Source: CAD feature listing. Evaluate the final solid. Frame: model axes, mm. A direction names the side the tool comes from. Give positions to 0.01 mm unless a question says otherwise; leave off trailing zeros. Loops run counter-clockwise (first coordinate to the right, second up) from the corner with the lowest first, then second, coordinate; pieces in that order, holes last. Notation, with made-up numbers: M 14,-31 L 25,-31 A24 cw 25,6 Z; hole C 35,-32 d2. An arc over 180 degrees is marked long. Answer in a Markdown table with one row per item.
```python
from build123d import *

# Parameters (mm, degrees)
F0_W     = 10
F0_H     = 75
F1_DEPTH = 12.5
F2_R     = 5
F3_DEPTH = 400.001
F4_R     = 5
F5_DEPTH = 50
F6_R     = 20
F7_R     = 3
F8_DEPTH = 140.9584442942


with BuildPart() as f1:
    # F0 (on Front) → F1 (new body, symmetric)
    with BuildSketch(Plane.XZ):
        Polygon((129.7779953739, 41.1399305532), (-70.2220046261, 41.1399305532), (-70.2220046261, 25.182486259), (-60.2220046261, 25.182486259), (129.7779953739, 25.182486259), align=None)
        Polygon((329.7779953739, 41.1399305532), (129.7779953739, 41.1399305532), (129.7779953739, 25.182486259), (319.7779953739, 25.182486259), (329.7779953739, 25.182486259), align=None)
        with Locations((-65.2220046261, -12.317513741)):
            Rectangle(F0_W, F0_H)
        with Locations((324.7779953739, -12.317513741)):
            Rectangle(F0_W, F0_H)
    extrude(amount=F1_DEPTH, both=True)

    # F2 (on face) → F3 (cut, through all)
    with BuildSketch(Plane(origin=(-70.2220046261, 0, 0), x_dir=(0, -1, 0), z_dir=(-1, 0, 0))):
        with Locations((0, -29.817513741)):
            Circle(F2_R)
    extrude(amount=-F3_DEPTH, mode=Mode.SUBTRACT)

    # F4 (on face) → F5 (join)
    with BuildSketch(Plane.XY.offset(41.1399305532)):
        with Locations((129.7779953739, 0)):
            Circle(F4_R)
    extrude(amount=F5_DEPTH)

    # F6
    f6_edges = [f1.edges().sort_by_distance(p)[0] for p in [
        (-60.222005, 0, 25.182486),
        (319.777995, 0, 25.182486),
    ]]
    fillet(f6_edges, radius=F6_R)

    # F7 (on face) → F8 (cut, through all)
    with BuildSketch(Plane.XY.offset(91.1399305532)):
        with Locations((129.7779953739, 0)):
            Circle(F7_R)
    extrude(amount=-F8_DEPTH, mode=Mode.SUBTRACT)


solid = f1.part
```
1) Set-up query: faces 4 (the flat face through (127, -3, 25.182)), 5 (the cylindrical face through (134.547, 1.502, 65.79)), 6 (the flat face through (129.7, -3.3, 91.14)). Return all of +Z, -Z, +X, -X, +Y, -Y with unobstructed straight access to the full face (end or side cutting, diameter ignored); none if empty.
Reply:
| item | result |
|---|---|
| face 4 | -Z, +Y, -Y |
| face 5 | +Z |
| face 6 | +Z, +X, -X, +Y, -Y |
2) Pull-direction query (Z, two-part tool) for faces 1 (the cylindrical face through (324.71, 1.08, -34.7)), 2 (the flat face through (-60.222, 0, -23)), 3 (the flat face through (133, -6, 41.14)); classes: released by +Z, released by -Z, zero draft, split by the parting line, or undercut.
Reply:
| item | result |
|---|---|
| face 1 | undercut |
| face 2 | zero draft |
| face 3 | released by +Z |
3) Pin query (flat end, axial travel): pin 1 Ø7.5 at (x, y) = (46, -5) entering from -Z; pin 2 Ø12 at (x, y) = (288, -9) entering from +Z. Return the tip coordinate at first contact, or that it passes through.
Reply:
| item | result |
|---|---|
| pin 1 | stops at z = 25.18 |
| pin 2 | stops at z = 41.14 |
4) Section B-B, the plane x = 231. Return loops of the section in (y, z).
Reply:
| item | result |
|---|---|
| outline | M -12.5,25.18 L 12.5,25.18 L 12.5,41.14 L -12.5,41.14 Z |
5) Section C-C, the plane z = 75. Return loops of the section in (x, y), then the cut area to 3 significant figures.
Reply:
| item | result |
|---|---|
| outline | C 129.78,0 d10; hole C 129.78,0 d6 |
| area | 50.3 mm² |
6) Material intervals for L1, parallel to X at y = -11.25, z = -35.5; L2, parallel to Z at x = 326.25, y = 0; L3, parallel to Z at x = 210, y = -0.25, sorted ascending.
Reply:
| item | result |
|---|---|
| L1 | x = -70.22 to -60.22, 319.78 to 329.78 |
| L2 | z = -49.82 to -34.82, -24.82 to 41.14 |
| L3 | z = 25.18 to 41.14 |
7) Section A-A, the plane z = -20. Return loops of the section in (x, y).
Reply:
| item | result |
|---|---|
| outline | M -70.22,-12.5 L -60.22,-12.5 L -60.22,12.5 L -70.22,12.5 Z; M 319.78,-12.5 L 329.78,-12.5 L 329.78,12.5 L 319.78,12.5 Z |
